```python
from build123d import *

# Parameters (mm, degrees)
SKETCH_1_W      = 170
SKETCH_1_H      = 105
SKETCH_1_R      = 2
SKETCH_1_R_2    = 1.5
EXTRUDE_1_DEPTH = 5


with BuildPart() as part:
    # ｽｹｯﾁ1 → ﾎﾞｽ - 押し出し1 (new body)
    with BuildSketch(Plane(origin=(0, 0, 0), x_dir=(1, 0, 0), z_dir=(0, 1, 0))):
        with Locations((85, 52.5)):
            Rectangle(SKETCH_1_W, SKETCH_1_H)
        with Locations((11, 94)):
            Circle(SKETCH_1_R, mode=Mode.SUBTRACT)
        with Locations((11, 11)):
            Circle(SKETCH_1_R, mode=Mode.SUBTRACT)
        with Locations((159, 11)):
            Circle(SKETCH_1_R, mode=Mode.SUBTRACT)
        with Locations((159, 94)):
            Circle(SKETCH_1_R, mode=Mode.SUBTRACT)
        with Locations((54.4, 12.5)):
            Circle(SKETCH_1_R_2, mode=Mode.SUBTRACT)
        with Locations((27.4, 12.5)):
            Circle(SKETCH_1_R_2, mode=Mode.SUBTRACT)
        with Locations((54.4, 32.5)):
            Circle(SKETCH_1_R_2, mode=Mode.SUBTRACT)
        with Locations((27.4, 32.5)):
            Circle(SKETCH_1_R_2, mode=Mode.SUBTRACT)
        with Locations((60.88, 80.73)):
            Circle(SKETCH_1_R_2, mode=Mode.SUBTRACT)
        with Locations((65.97, 28.66)):
            Circle(SKETCH_1_R_2, mode=Mode.SUBTRACT)
        with Locations((93.92, 28.66)):
            Circle(SKETCH_1_R_2, mode=Mode.SUBTRACT)
        with Locations((109.12, 79.45)):
            Circle(SKETCH_1_R_2, mode=Mode.SUBTRACT)
        with Locations((115.6, 34.5)):
            Circle(SKETCH_1_R_2, mode=Mode.SUBTRACT)
        with Locations((142.6, 34.5)):
            Circle(SKETCH_1_R_2, mode=Mode.SUBTRACT)
        with Locations((142.6, 14.5)):
            Circle(SKETCH_1_R_2, mode=Mode.SUBTRACT)
        with Locations((115.6, 14.5)):
            Circle(SKETCH_1_R_2, mode=Mode.SUBTRACT)
    extrude(amount=EXTRUDE_1_DEPTH)


solid = part.part
```
Verification items for the finished model (mm, model axes). Coordinates: 2 decimals unless noted, no trailing zeros. Loops run counter-clockwise (first coordinate to the right, second up) from the corner with the lowest first, then second, coordinate; pieces in that order, holes last. Notation, with made-up numbers: (-9, 89) - (48, 89) arc R20 cw to (48, 100) - close; hole circle Ø3 at (-1, 67). An arc over 180 degrees is marked (long way). Put each result on its own line as item: value.
Item 1: Section check A-A (z = -94). Enter the section's corners in (x, y).
Conclusion:
outline: (0, 0) - (9, 0) - (9, 5) - (0, 5) - close; (13, 0) - (157, 0) - (157, 5) - (13, 5) - close; (161, 0) - (170, 0) - (170, 5) - (161, 5) - close
Item 2: Draft check along X on faces 1 (the face through (94.61, 2.46, -27.33)), 2 (the face through (84, 0, -53)), 3 (the face through (117.03, 2.46, -14.95)). Enter one of: pulls with the +X half, pulls with the -X half, needs draft (parallel to the pull), parting line crosses it, or undercut.
Conclusion:
face 1: undercut
face 2: needs draft
face 3: undercut
Item 3: Scan lines: line 1 along Z through (x, y) = (54.4, 2.45); line 2 along Z through (x, y) = (159, 1.3); line 3 along X through (y, z) = (2.8, -29). Record each from-to range of solid material in increasing order.
Conclusion:
line 1: z = -105 to -34, -31 to -14, -11 to 0
line 2: z = -105 to -96, -92 to -13, -9 to 0
line 3: x = 0 to 64.51, 67.43 to 92.46, 95.38 to 170
